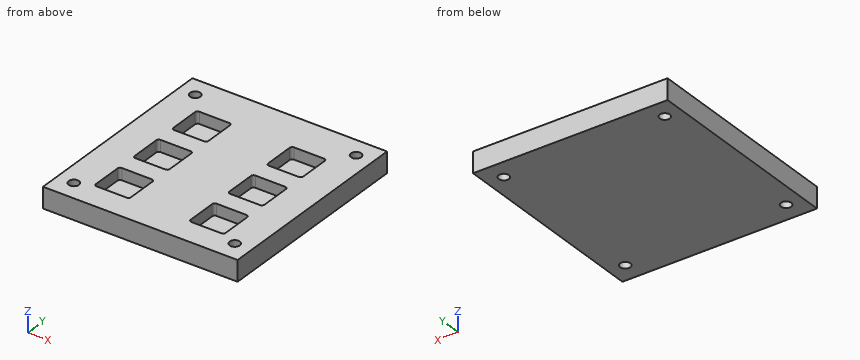
```python
from build123d import *

# Parameters (mm, degrees)
SKETCH1_W           = 150
SKETCH1_H           = 160
BOSS_EXTRUDE1_DEPTH = 16
CUT_EXTRUDE1_DEPTH  = 9
SKETCH3_R           = 4
CUT_EXTRUDE2_DEPTH  = 17


with BuildPart() as part:
    # Sketch1 → Boss-Extrude1 (new body)
    with BuildSketch(Plane.XY):
        Rectangle(SKETCH1_W, SKETCH1_H)
    extrude(amount=BOSS_EXTRUDE1_DEPTH)

    # Sketch2 → Cut-Extrude1 (cut)
    with BuildSketch(Plane.XY.offset(16)):
        with BuildLine():
            Line((-48, 23), (-25, 23))
            ThreePointArc((-25, 23), (-23.585786438, 23.585786438), (-23, 25))
            Line((-23, 25), (-23, 48))
            ThreePointArc((-23, 48), (-23.585786438, 49.414213562), (-25, 50))
            Line((-25, 50), (-48, 50))
            ThreePointArc((-48, 50), (-49.414213562, 49.414213562), (-50, 48))
            Line((-50, 48), (-50, 25))
            ThreePointArc((-50, 25), (-49.414213562, 23.585786438), (-48, 23))
        make_face()
        with BuildLine():
            Line((23, 25), (23, 48))
            ThreePointArc((23, 48), (23.585786438, 49.414213562), (25, 50))
            Line((25, 50), (48, 50))
            ThreePointArc((48, 50), (49.414213562, 49.414213562), (50, 48))
            Line((50, 48), (50, 25))
            ThreePointArc((50, 25), (49.414213562, 23.585786438), (48, 23))
            Line((48, 23), (25, 23))
            ThreePointArc((25, 23), (23.585786438, 23.585786438), (23, 25))
        make_face()
        with BuildLine():
            Line((-48, -60), (-25, -60))
            ThreePointArc((-25, -60), (-23.585786438, -59.414213562), (-23, -58))
            Line((-23, -58), (-23, -35))
            ThreePointArc((-23, -35), (-23.585786438, -33.585786438), (-25, -33))
            Line((-25, -33), (-48, -33))
            ThreePointArc((-48, -33), (-49.414213562, -33.585786438), (-50, -35))
            Line((-50, -35), (-50, -58))
            ThreePointArc((-50, -58), (-49.414213562, -59.414213562), (-48, -60))
        make_face()
        with BuildLine():
            Line((23, -58), (23, -35))
            ThreePointArc((23, -35), (23.585786438, -33.585786438), (25, -33))
            Line((25, -33), (48, -33))
            ThreePointArc((48, -33), (49.414213562, -33.585786438), (50, -35))
            Line((50, -35), (50, -58))
            ThreePointArc((50, -58), (49.414213562, -59.414213562), (48, -60))
            Line((48, -60), (25, -60))
            ThreePointArc((25, -60), (23.585786438, -59.414213562), (23, -58))
        make_face()
        with BuildLine():
            Line((-25, -18.5), (-48, -18.5))
            ThreePointArc((-48, -18.5), (-49.414213562, -17.914213562), (-50, -16.5))
            Line((-50, -16.5), (-50, 6.5))
            ThreePointArc((-50, 6.5), (-49.414213562, 7.914213562), (-48, 8.5))
            Line((-48, 8.5), (-25, 8.5))
            ThreePointArc((-25, 8.5), (-23.585786438, 7.914213562), (-23, 6.5))
            Line((-23, 6.5), (-23, -16.5))
            ThreePointArc((-23, -16.5), (-23.585786438, -17.914213562), (-25, -18.5))
        make_face()
        with BuildLine():
            Line((50, -16.5), (50, 6.5))
            ThreePointArc((50, 6.5), (49.414213562, 7.914213562), (48, 8.5))
            Line((48, 8.5), (25, 8.5))
            ThreePointArc((25, 8.5), (23.585786438, 7.914213562), (23, 6.5))
            Line((23, 6.5), (23, -16.5))
            ThreePointArc((23, -16.5), (23.585786438, -17.914213562), (25, -18.5))
            Line((25, -18.5), (48, -18.5))
            ThreePointArc((48, -18.5), (49.414213562, -17.914213562), (50, -16.5))
        make_face()
    extrude(amount=-CUT_EXTRUDE1_DEPTH, mode=Mode.SUBTRACT)

    # Sketch3 → Cut-Extrude2 (cut, through all)
    with BuildSketch(Plane.XY.offset(16)):
        with Locations((-62, 65)):
            Circle(SKETCH3_R)
        with Locations((62, 65)):
            Circle(SKETCH3_R)
        with Locations((62, -65)):
            Circle(SKETCH3_R)
        with Locations((-62, -65)):
            Circle(SKETCH3_R)
    extrude(amount=-CUT_EXTRUDE2_DEPTH, mode=Mode.SUBTRACT)


solid = part.part
```
Input: part model. Units: mm. Frame: model coordinates. Round coordinates to 2 decimals unless told otherwise and drop trailing zeros. Loops run counter-clockwise (first coordinate to the right, second up) from the corner with the lowest first, then second, coordinate; pieces in that order, holes last. Notation, with made-up numbers: (66.25, 13) -> (125.25, 13) arc R14 cw to (125.25, 33) -> close; hole circle Ø4 at (-18, 8). An arc over 180 degrees is marked (long way). One line per item, written item: value.
(1) Section D-D (x = -28). Return the cut outline in (y, z), plus the area to 3 significant figures.
Geometry check:
outline: (-80, 0) -> (80, 0) -> (80, 16) -> (50, 16) -> (50, 7) -> (23, 7) -> (23, 16) -> (8.5, 16) -> (8.5, 7) -> (-18.5, 7) -> (-18.5, 16) -> (-33, 16) -> (-33, 7) -> (-60, 7) -> (-60, 16) -> (-80, 16) -> close
area: 1,830 mm2
(2) Section A-A (x = -62). Return the cut outline in (y, z).
Geometry check:
outline: (-80, 0) -> (-69, 0) -> (-69, 16) -> (-80, 16) -> close; (-61, 0) -> (61, 0) -> (61, 16) -> (-61, 16) -> close; (69, 0) -> (80, 0) -> (80, 16) -> (69, 16) -> close
(3) Section B-B (y = -65). Return the cut outline in (x, z), plus the area to 3 significant figures.
Geometry check:
outline: (-75, 0) -> (-66, 0) -> (-66, 16) -> (-75, 16) -> close; (-58, 0) -> (58, 0) -> (58, 16) -> (-58, 16) -> close; (66, 0) -> (75, 0) -> (75, 16) -> (66, 16) -> close
area: 2,140 mm2
(4) Section C-C (z = 12.75). Give the number of separate pieces and of enclosed holes in the cut face, plus the area to 3 significant figures.
Geometry check:
separate pieces: 1
enclosed holes: 10
area: 19,400 mm2
(5) Material intervals for line 1 (Y direction, x = -42, z = 12.5); line 2 (Y direction, x = 62, z = 11.75); line 3 (X direction, y = -65.5, z = 11.75), sorted ascending. Write a range as [from, to].
Geometry check:
line 1: [-80, -60], [-33, -18.5], [8.5, 23], [50, 80]
line 2: [-80, -69], [-61, 61], [69, 80]
line 3: [-75, -65.97], [-58.03, 58.03], [65.97, 75]
